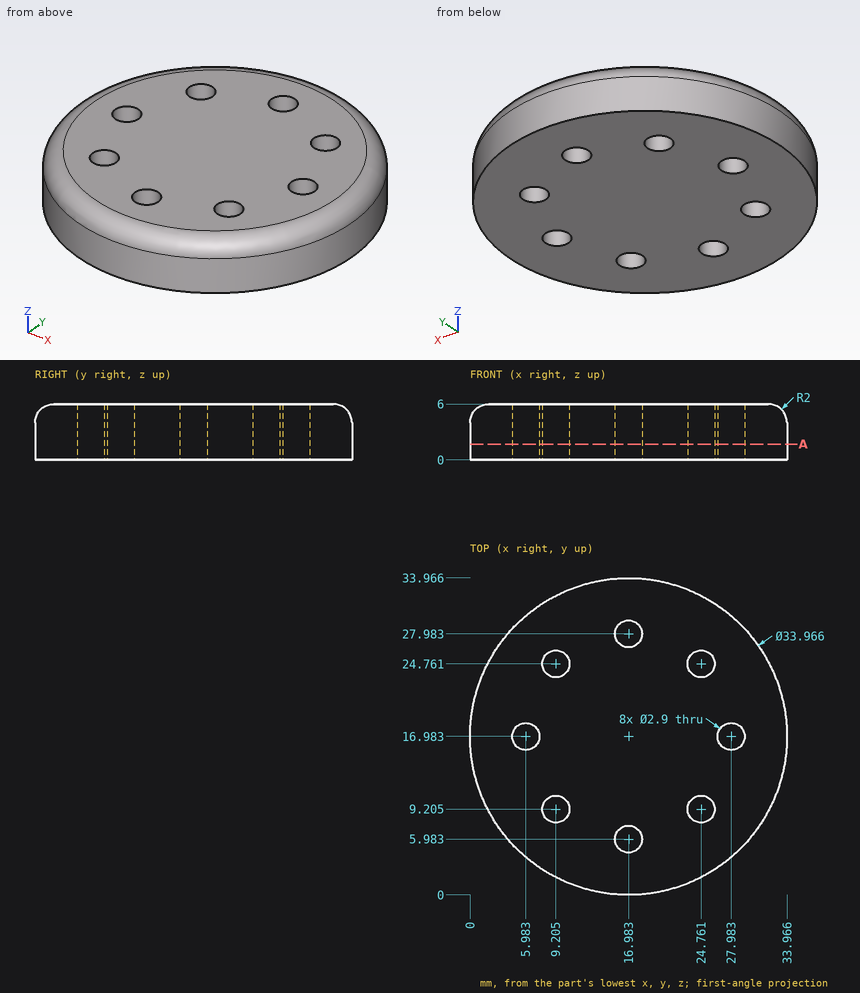
Verification items for this drawing (mm, ordinates from the low corner). Round coordinates to 2 decimals unless told otherwise and drop trailing zeros. Write item = value, one per line. Start each with the question number.
1) Sectioned sample at A-A, the plane z = 1.7. State how many separate pieces and enclosed holes the cut face has, plus the area to 3 significant figures.
2) Gauge pin test, flat ends, axial feed: pin 1 Ø1.5 at (x, z) = (4.5, 1) entering from -Y (1 decimal); pin 2 Ø2.5 at (x, y) = (16.98, 5.98) entering from -Z; pin 3 Ø1.5 at (x, z) = (13, 1) entering from -Y; pin 4 Ø2 at (y, z) = (15, 2.5) entering from +X. Record the tip position at first contact, or that the pin passes through.
3) Thickness scan on probe 1 along Y at (x, z) = (24.5, 1.3) (1 decimal); probe 2 along Y at (x, z) = (8.5, 2.8) (1 decimal); probe 3 along Y at (x, z) = (6, 5.7) (1 decimal). Record the ranges inside material, lowest first.
Results are:
q1.separate_pieces = 1
q1.enclosed_holes = 8
q1.area = 853 mm^2
q2.pin_1 = 4.7
q2.pin_2 = through
q2.pin_3 = 0.31
q2.pin_4 = 33.94
q3.probe_1 = 1.8 to 7.8, 10.6 to 23.3, 26.2 to 32.2
q3.probe_2 = 2.3 to 7.9, 10.5 to 23.5, 26 to 31.7
q3.probe_3 = 5.3 to 15.5, 18.4 to 28.7
